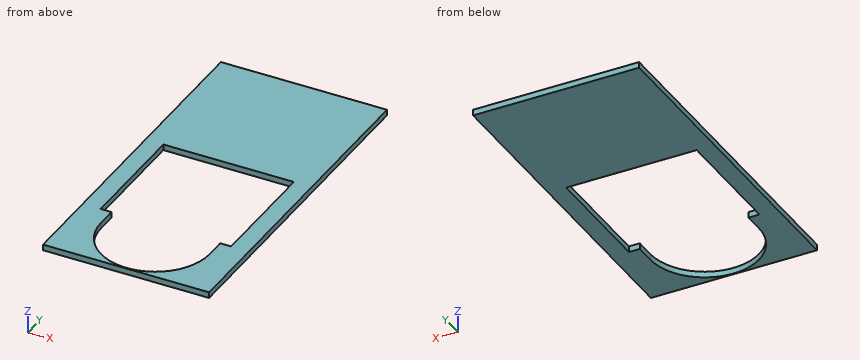
from build123d import *

# Parameters (mm, degrees)
SKETCH_1_W          = 84
SKETCH_1_H          = 170
EXTRUDE_1_DEPTH     = 3
SKETCH_2_R          = 27.5
SKETCH_2_W          = 66
SKETCH_2_H          = 60
CUT_EXTRUDE_1_DEPTH = 3


with BuildPart() as part:
    # Sketch 1 → Extrude 1 (new body)
    with BuildSketch(Plane.XY):
        with Locations((42, 85)):
            Rectangle(SKETCH_1_W, SKETCH_1_H)
    extrude(amount=EXTRUDE_1_DEPTH)

    # Sketch 2 → Cut-Extrude 1 (cut)
    with BuildSketch(Plane.XY.offset(3)):
        with Locations((42, 28)):
            Circle(SKETCH_2_R)
        with Locations((42, 68)):
            Rectangle(SKETCH_2_W, SKETCH_2_H)
        with BuildLine():
            ThreePointArc((67.617376915, 38), (42, 55.5), (16.382623085, 38))
            Line((16.382623085, 38), (67.617376915, 38))
        make_face()
        with BuildLine():
            Line((14.5, 59.117124135), (14.5, 38))
            Line((14.5, 38), (16.382623085, 38))
            ThreePointArc((16.382623085, 38), (42, 55.5), (67.617376915, 38))
            Line((67.617376915, 38), (69.5, 38))
            Line((69.5, 38), (69.5, 59.117124135))
            Line((69.5, 59.117124135), (14.5, 59.117124135))
        make_face()
        with BuildLine():
            Line((16.382623085, 38), (14.5, 38))
            Line((14.5, 38), (14.5, 28))
            ThreePointArc((14.5, 28), (14.974753792, 33.087835239), (16.382623085, 38))
        make_face()
        with BuildLine():
            Line((69.5, 28), (69.5, 38))
            Line((69.5, 38), (67.617376915, 38))
            ThreePointArc((67.617376915, 38), (69.025246208, 33.087835239), (69.5, 28))
        make_face()
        with BuildLine():
            Line((69.5, 28), (14.5, 28))
            ThreePointArc((14.5, 28), (42, 0.5), (69.5, 28))
        make_face()
    extrude(amount=-CUT_EXTRUDE_1_DEPTH, mode=Mode.SUBTRACT)


solid = part.part
Model file for the job. Use its own axes, mm. Give positions to 0.01 mm unless a question says otherwise; leave off trailing zeros. Order: outer loops, then holes, each group sorted by start corner. A loop starts at its lowest first (then second) coordinate and runs counter-clockwise, first axis right, second up. Notation, with made-up numbers: (-30.5, -17.75) - (-6.5, -17.75) arc R26 cw to (-6.5, 14.25) - close; hole circle Ø11 at (47, 72.5). An arc over 180 degrees is marked (long way). One line per item, written item: value.
Item 1: Slice it at B-B (y = 32). List the corners of the cut face in (x, z).
Response values:
outline: (0, 0) - (14.5, 0) - (14.5, 3) - (0, 3) - close; (69.5, 0) - (84, 0) - (84, 3) - (69.5, 3) - close
Item 2: Slice it at C-C (z = 2.1). List the corners of the cut face in (x, y), then the cut area to 3 significant figures.
Response values:
outline: (0, 0) - (84, 0) - (84, 170) - (0, 170) - close; hole (9, 38) - (14.5, 38) - (14.5, 28) arc R27.5 ccw to (69.5, 28) - (69.5, 38) - (75, 38) - (75, 98) - (9, 98) - close
area: 8,580 mm2
Item 3: Slice it at A-A (x = 42). List the corners of the cut face in (y, z).
Response values:
outline: (0, 0) - (0.5, 0) - (0.5, 3) - (0, 3) - close; (98, 0) - (170, 0) - (170, 3) - (98, 3) - close
Item 4: Wall check: line 1 (X direction, y = 69.5, z = 1.85); line 2 (Y direction, x = 10.5, z = 1.15); line 3 (Y direction, x = 45, z = 2.7). Give the ranges that are in metal, low to high.
Response values:
line 1: 0 to 9, 75 to 84
line 2: 0 to 38, 98 to 170
line 3: 0 to 0.66, 98 to 170
